```python
from build123d import *

# Parameters (mm, degrees)
SKETCH_1_W          = 10
SKETCH_1_H          = 10
SKETCH_1_W_2        = 8
SKETCH_1_H_2        = 8
EXTRUDE_1_DEPTH     = 513.21590794
SKETCH_4_R          = 2.15
CUT_EXTRUDE_2_DEPTH = 514.337674599


with BuildPart() as part:
    # ｽｹｯﾁ1 → 押し出し-薄板1 (new body)
    with BuildSketch(Plane(origin=(0, 0, 0), x_dir=(1, 0, 0), z_dir=(0, 1, 0))):
        Rectangle(SKETCH_1_W, SKETCH_1_H)
        Rectangle(SKETCH_1_W_2, SKETCH_1_H_2, mode=Mode.SUBTRACT)
    extrude(amount=EXTRUDE_1_DEPTH)

    # ｽｹｯﾁ4 → ｶｯﾄ - 押し出し2 (cut, through all)
    with BuildSketch(Plane.ZY.offset(-5)):
        with Locations(Location((0, 508.21590794, 0), (0, 0, 180))):
            Circle(SKETCH_4_R)
        with Locations(Location((0, 5, 0), (0, 0, 180))):
            Circle(SKETCH_4_R)
    extrude(amount=CUT_EXTRUDE_2_DEPTH, mode=Mode.SUBTRACT)


solid = part.part
```
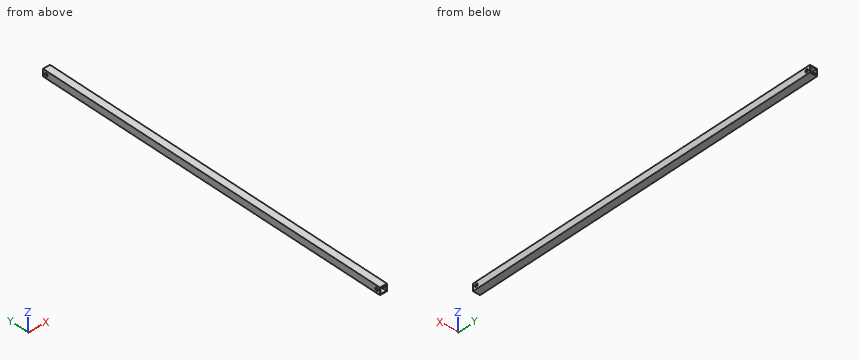
Can you work these out from the model? Positions are in its coordinate system, mm. Round coordinates to 2 decimals unless told otherwise and drop trailing zeros. Loops run counter-clockwise (first coordinate to the right, second up) from the corner with the lowest first, then second, coordinate; pieces in that order, holes last. Notation, with made-up numbers: (68, 5) -> (81, 5) arc R16 cw to (81, 12) -> close; hole circle Ø6 at (-37.5, -31). An arc over 180 degrees is marked (long way). One line per item, written item: value. Start each with the question number.
1. If I drill on probe 1 along Y at (x, z) = (-4.6, 0); probe 2 along Z at (x, y) = (1, 308), over which ranges is the centre line in solid material (lowest first)?
2. If we section it at B-B, the plane z = 0: Write out the boundary of the cut face in (x, y).
3. If we section it at C-C, the plane y = 371: Write out the boundary of the cut face in (x, z), then the cut area to 3 significant figures.
4. If we section it at A-A, the plane x = -0.25: Write out the boundary of the cut face in (y, z), then the cut area to 3 significant figures.
5. For pin 1 (2.5 mm diameter, centred on y = 508.22, z = 0, fed in from +X); pin 2 (5.5 mm diameter, centred on y = 5, z = 0, fed in from +X), each with a flat end and sliding along its axis, tell me the tip position at first contact or that it passes through.
Calculated:
1. probe 1: y = 0 to 2.85, 7.15 to 506.07, 510.37 to 513.22
1. probe 2: z = -5 to -4, 4 to 5
2. outline: (-5, 0) -> (-4, 0) -> (-4, 2.85) -> (-5, 2.85) -> close; (-5, 7.15) -> (-4, 7.15) -> (-4, 506.07) -> (-5, 506.07) -> close; (-5, 510.37) -> (-4, 510.37) -> (-4, 513.22) -> (-5, 513.22) -> close; (4, 0) -> (5, 0) -> (5, 2.85) -> (4, 2.85) -> close; (4, 7.15) -> (5, 7.15) -> (5, 506.07) -> (4, 506.07) -> close; (4, 510.37) -> (5, 510.37) -> (5, 513.22) -> (4, 513.22) -> close
3. outline: (-5, -5) -> (5, -5) -> (5, 5) -> (-5, 5) -> close; hole (-4, -4) -> (4, -4) -> (4, 4) -> (-4, 4) -> close
3. area: 36.0 mm²
4. outline: (0, -5) -> (513.22, -5) -> (513.22, -4) -> (0, -4) -> close; (0, 4) -> (513.22, 4) -> (513.22, 5) -> (0, 5) -> close
4. area: 1,030 mm²
5. pin 1: passes through
5. pin 2: stops at x = 5
